Autodesk Inventor part; units mm, degrees
ref_plane "工作平面1" through (0, 0, 42) normal (0, 0, 1) x (1, 0, 0)
ref_plane "YZ Plane" through (0, 0, 0) normal (1, 0, 0) x (0, 1, 0)
ref_plane "XZ Plane" through (0, 0, 0) normal (0, 1, 0) x (-1, 0, 0)
ref_plane "工作平面1" through (0, 0, 42) normal (0, 0, 1) x (1, 0, 0)
sketch "草图1" plane through (0, 0, 42) normal (0, 0, 1) x (1, 0, 0)
  line L0 (0, 0) -> (60, 0)
  line L1 (60, 0) -> (60, -1169.8)
  line L2 (60, -1169.8) -> (0, -1169.8)
  line L3 (0, -1169.8) -> (0, 0)
  line L4 (0, -80.6) -> (60, -80.6)
  line L5 (0, -191.9) -> (60, -191.9)
  line L6 (0, -276.5) -> (60, -276.5)
  line L7 (0, -335.9) -> (60, -335.9)
  line L8 (0, -420.6) -> (60, -420.6)
  line L9 (0, -550.6) -> (60, -550.6)
  line L10 (0, -677.8) -> (60, -677.8)
  line L11 (0, -782.9) -> (60, -782.9)
  line L12 (0, -839.5) -> (60, -839.5)
  line L13 (0, -923.6) -> (60, -923.6)
  line L14 (0, -1007.7) -> (60, -1007.7)
  line L15 (0, -1091.2) -> (60, -1091.2)
  line L16 (60, 0) -> (118.4, 0)
  line L17 (118.4, 0) -> (118.4, -23.7)
  line L18 (118.4, -23.7) -> (83.4, -23.7)
  line L19 (83.4, -23.7) -> (83.4, -79.7)
  line L20 (83.4, -79.7) -> (118.4, -79.7)
  line L21 (118.4, -79.7) -> (118.4, -137.6)
  line L22 (118.4, -137.6) -> (83.4, -137.6)
  line L23 (83.4, -137.6) -> (83.4, -276.5)
  line L24 (83.4, -276.5) -> (142.9, -276.5)
  line L25 (142.9, -276.5) -> (142.9, -379.5)
  line L26 (83.4, -276.5) -> (83.4, -379.5)
  line L27 (83.4, -379.5) -> (142.9, -379.5)
  line L28 (142.9, -379.5) -> (142.9, -463)
  line L29 (142.9, -463) -> (83.4, -463)
  line L30 (83.4, -463) -> (83.4, -379.5)
  line L31 (142.9, -463) -> (142.9, -566.2)
  line L32 (142.9, -566.2) -> (83.4, -566.2)
  line L33 (83.4, -566.2) -> (83.4, -463)
  line L34 (142.9, -566.2) -> (146.7, -566.2)
  line L35 (146.7, -566.2) -> (146.7, -616.2)
  line L36 (146.7, -616.2) -> (192.5, -616.2)
  line L37 (192.5, -616.2) -> (192.5, -673.2)
  line L38 (192.5, -616.2) -> (342.5, -616.2)
  line L39 (342.5, -616.2) -> (342.5, -673.2)
  line L40 (342.5, -673.2) -> (143.4, -673.2)
  line L41 (143.4, -673.2) -> (83.4, -673.2)
  line L42 (83.4, -673.2) -> (83.4, -1092.3)
  line L43 (83.4, -1092.3) -> (143.4, -1092.3)
  line L44 (143.4, -1092.3) -> (143.4, -673.2)
  line L45 (83.4, -754.3) -> (143.4, -754.3)
  line L46 (143.4, -837.8) -> (83.4, -837.8)
  line L47 (83.4, -893.6) -> (143.4, -893.6)
  line L48 (143.4, -978.3) -> (83.4, -978.3)
  line L49 (60, -1169.8) -> (188.1, -1169.8)
  line L50 (188.1, -1169.8) -> (188.1, -1092.3)
  line L51 (188.1, -1092.3) -> (143.4, -1092.3)
  line L52 (83.4, -1092.3) -> (83.4, -1117.3)
  line L53 (83.4, -1117.3) -> (188.1, -1117.3)
  line L54 (98.6, -1092.3) -> (98.6, -1117.3)
  line L55 (114.5, -1092.3) -> (114.5, -1117.3)
  line L56 (143.4, -1092.3) -> (143.4, -1117.3)
  line L57 (166.2, -1092.3) -> (166.2, -1117.3)
  line L58 (188.1, -1163.6) -> (336, -1163.6)
  line L59 (188.1, -1137.1) -> (336, -1137.1)
  line L60 (336, -1137.1) -> (336, -1163.6)
  dimension "d1" = 60
  dimension "d2" = 80.6
  dimension "d3" = 111.3
  dimension "d4" = 84.6
  dimension "d5" = 59.4
  dimension "d6" = 84.7
  dimension "d7" = 130
  dimension "d8" = 127.2
  dimension "d9" = 105.1
  dimension "d10" = 56.6
  dimension "d11" = 84.1
  dimension "d12" = 84.1
  dimension "d13" = 83.5
  dimension "d14" = 78.6
  dimension "d15" = 58.4
  dimension "d16" = 23.7
  dimension "d17" = 35
  dimension "d18" = 56
  dimension "d19" = 57.9
  dimension "d20" = 35
  dimension "d21" = 138.9
  dimension "d22" = 59.5
  dimension "d23" = 103
  dimension "d24" = 83.5
  dimension "d25" = 103.2
  dimension "d26" = 59.5
  dimension "d27" = 3.8
  dimension "d28" = 50
  dimension "d29" = 45.8
  dimension "d30" = 57
  dimension "d31" = 150
  dimension "d32" = 57
  dimension "d33" = 199.1
  dimension "d34" = 60
  dimension "d36" = 81.1
  dimension "d37" = 83.5
  dimension "d38" = 55.8
  dimension "d39" = 84.7
  dimension "d40" = 114
  dimension "d41" = 128.1
  dimension "d42" = 25
  dimension "d43" = 15.2
  dimension "d44" = 15.9
  dimension "d45" = 28.9
  dimension "d46" = 22.8
  dimension "d47" = 21.9
  dimension "d48" = 147.9
  dimension "d49" = 6.2
  dimension "d50" = 26.5
extrude "拉伸1" add sketch "草图1" against normal blind 1
properties part number "LabVIEWM0.5"
Check sheet for the modelled part. Datum: model origin and axes. Units: mm. Round coordinates to 2 decimals unless told otherwise and drop trailing zeros. Order: outer loops, then holes, each group sorted by start corner. A loop starts at its lowest first (then second) coordinate and runs counter-clockwise, first axis right, second up.
Q1. Scan lines: L1, parallel to Y at x = 186.5, z = 41.6; L2, parallel to Y at x = 194, z = 41.45; L3, parallel to Y at x = 125, z = 41.35. Record each from-to range of solid material in increasing order.
Filled sheet:
L1: y = -1169.8 to -1092.3, -673.2 to -616.2
L2: y = -1163.6 to -1137.1, -673.2 to -616.2
L3: y = -1169.8 to -276.5
Q2. Cross-section at C-C, the plane y = -872.5. Enter the section's corners in (x, z).
Filled sheet:
outline: (0, 41) - (143.4, 41) - (143.4, 42) - (0, 42) - close
Q3. Cross-section at A-A, the plane x = 273.5. Enter the section's corners in (y, z), plus the area to 3 significant figures.
Filled sheet:
outline: (-1163.6, 41) - (-1137.1, 41) - (-1137.1, 42) - (-1163.6, 42) - close; (-673.2, 41) - (-616.2, 41) - (-616.2, 42) - (-673.2, 42) - close
area: 83.5 mm2
Q4. Depth check by flat-ended pin: P1, Ø0.5, axis at x = 144.5, z = 41.5, coming from the +Y side; P2, Ø0.5, axis at x = 234, z = 41.5, coming from the -Y side; P3, Ø0.5, axis at y = -880, z = 41.5, coming from the +X side. Enter the tip coordinate at first touch or a pass-through.
Filled sheet:
P1: stops at y = -566.2
P2: stops at y = -1163.6
P3: stops at x = 143.4
Q5. Cross-section at D-D, the plane y = -193. Enter the section's corners in (x, z).
Filled sheet:
outline: (0, 41) - (83.4, 41) - (83.4, 42) - (0, 42) - close
Q6. Cross-section at B-B, the plane z = 41.75. Enter the section's corners in (x, y), plus the area to 3 significant figures.
Filled sheet:
outline: (0, -1169.8) - (188.1, -1169.8) - (188.1, -1163.6) - (336, -1163.6) - (336, -1137.1) - (188.1, -1137.1) - (188.1, -1092.3) - (143.4, -1092.3) - (143.4, -673.2) - (342.5, -673.2) - (342.5, -616.2) - (146.7, -616.2) - (146.7, -566.2) - (142.9, -566.2) - (142.9, -276.5) - (83.4, -276.5) - (83.4, -137.6) - (118.4, -137.6) - (118.4, -79.7) - (83.4, -79.7) - (83.4, -23.7) - (118.4, -23.7) - (118.4, 0) - (0, 0) - close
area: 173,000 mm2
